Read the model definition and answer for the solid it produces. Units are mm, in the model's axes. A direction names the side the tool comes from. Coordinates: 2 decimals unless noted, no trailing zeros. Loops run counter-clockwise (first coordinate to the right, second up) from the corner with the lowest first, then second, coordinate; pieces in that order, holes last. Notation, with made-up numbers: (89, 7) - (119, 7) arc R23 ccw to (119, 17) - close; hole circle Ø6 at (53.5, -19.5). An arc over 180 degrees is marked (long way). Use one line per item in the form item = value. Start each with the question number.
1) A cutting plane is placed at D-D (y = -2.25). Give the vertices of the cut face in (x, z), and give its area (3 significant figures).
2) Which of the six approach directions +Z, -Z, +X, -X, +Y, -Y give full straight-line access (tool end or side, diameter ignored) to faces 4 (the face through (0.1, -9.9, 6.1)), 5 (the face through (15, -10, 0)), 6 (the face through (12.37, -8.606, -9.014)), 7 (the face through (11.2, -11.2, 7))?
3) A cutting plane is placed at B-B (x = 10). Give the vertices of the cut face in (y, z), and give its area (4 significant figures).
4) The mould has two halves that part along Y. Classify faces 1 (the face through (8, -20, -2)), 2 (the face through (7.61, -8.64, -9.01)), 3 (the face through (-6.97, -9.86, -7.17)): released by +Y, released by -Y, zero draft, split by the parting line, or undercut.
5) Consider line 1 (Y direction, x = 10, z = -2.75); line 2 (X direction, y = -10, z = -3); line 3 (Z direction, x = -8, y = -6.5). Determine where each line is inside the solid, lowest interval first.
6) A cutting plane is placed at A-A (z = 2.5). Give the vertices of the cut face in (x, y), and give its area (3 significant figures).
7) Each of these flat-tipped pins is pushed along its axis until it touches: P1, Ø1.6, axis at x = 10, z = -9, coming from the +Y side; P2, Ø1.6, axis at x = 10.5, y = -11, coming from the +Z side; P3, Ø2, axis at x = 24, y = -12, coming from the -Z side; P4, Ø3, axis at x = -8.5, y = -6.5, coming from the -Z side. Where does it stop, or does it pass through?
8) A cutting plane is placed at C-C (x = 1). Give the vertices of the cut face in (y, z).
from build123d import *

# Parameters (mm, degrees)
F0_R      = 6.1
F1_DEPTH  = 20
F3_R      = 1.5
F4_DEPTH  = 25
F5_DEPTH  = 25
F6_R      = 5
F7_DEPTH  = 10
F8_R      = 2.75
F8_R_2    = 1.5
F9_DEPTH  = 3
F10_R     = 1.5
F11_DEPTH = 2


with BuildPart() as f1:
    # F0 (on Front) → F1 (new body)
    with BuildSketch(Plane.XZ):
        with BuildLine():
            ThreePointArc((0, 10), (7.0710678119, 7.0710678119), (10, 0))
            ThreePointArc((10, 0), (7.0710678119, -7.0710678119), (0, -10))
            Line((0, -10), (20, -10))
            Line((20, -10), (20, 10))
            Line((20, 10), (0, 10))
        make_face()
        with BuildLine():
            ThreePointArc((0, -10), (7.0710678119, -7.0710678119), (10, 0))
            ThreePointArc((10, 0), (7.0710678119, 7.0710678119), (0, 10))
            ThreePointArc((0, 10), (-10, 0), (0, -10))
        make_face()
        Circle(F0_R, mode=Mode.SUBTRACT)
    extrude(amount=F1_DEPTH)

    # F3 (on face) → F4 (cut)
    with BuildSketch(Plane.XY.offset(10)):
        with Locations((10, -10)):
            Circle(F3_R)
    extrude(amount=-F4_DEPTH, mode=Mode.SUBTRACT)

    # F2 (on face) → F5 (cut)
    with BuildSketch(Plane.XZ.offset(20)):
        with BuildLine():
            Line((-9.9874921777, 0.5), (-17.8410350345, 0.5))
            Line((-17.8410350345, 0.5), (-17.8410350345, -0.5))
            Line((-17.8410350345, -0.5), (-9.9874921777, -0.5))
            ThreePointArc((-9.9874921777, -0.5), (-10, 0), (-9.9874921777, 0.5))
        make_face()
        with BuildLine():
            Line((-6.0794736614, 0.5), (-9.9874921777, 0.5))
            ThreePointArc((-9.9874921777, 0.5), (-10, 0), (-9.9874921777, -0.5))
            Line((-9.9874921777, -0.5), (-6.0794736614, -0.5))
            ThreePointArc((-6.0794736614, -0.5), (-6.1, 0), (-6.0794736614, 0.5))
        make_face()
        with BuildLine():
            Line((15, 0.5), (6.0794736614, 0.5))
            ThreePointArc((6.0794736614, 0.5), (6.0948662551, 0.2502105766), (6.1, 0))
            ThreePointArc((6.1, 0), (6.0948662551, -0.2502105766), (6.0794736614, -0.5))
            Line((6.0794736614, -0.5), (15, -0.5))
            Line((15, -0.5), (15, 0.5))
        make_face()
    extrude(amount=-F5_DEPTH, mode=Mode.SUBTRACT)

    # F6 (on face) → F7 (join)
    with BuildSketch(Plane.YZ.offset(20)):
        with Locations((-10, 0)):
            Circle(F6_R)
    extrude(amount=F7_DEPTH)

    # F8 (on face) → F9 (cut)
    with BuildSketch(Plane.XY.offset(10)):
        with Locations((10, -10)):
            Circle(F8_R)
        with Locations((10, -10)):
            Circle(F8_R_2, mode=Mode.SUBTRACT)
    extrude(amount=-F9_DEPTH, mode=Mode.SUBTRACT)

    # F10 (on face) → F11 (cut)
    with BuildSketch(Plane(origin=(0, 0, -10), x_dir=(1, 0, 0), z_dir=(0, 0, -1))):
        Polygon((11.5877132403, 12.75), (8.4122867597, 12.75), (6.8245735195, 10), (8.4122867597, 7.25), (11.5877132403, 7.25), (13.1754264805, 10), align=None)
        with Locations((10, 10)):
            Circle(F10_R, mode=Mode.SUBTRACT)
    extrude(amount=-F11_DEPTH, mode=Mode.SUBTRACT)


solid = f1.part
Found:
q1.outline = (-9.99, -0.5) arc R10 ccw to (0, -10) - (20, -10) - (20, 10) - (0, 10) arc R10 ccw to (-9.99, 0.5) - (-6.08, 0.5) arc R6.1 cw to (6.08, 0.5) - (15, 0.5) - (15, -0.5) - (6.08, -0.5) arc R6.1 cw to (-6.08, -0.5) - close
q1.area = 427 mm^2
q2.face_4 = +Y, -Y
q2.face_5 = -X, +Y, -Y
q2.face_6 = -Z
q2.face_7 = +Z
q3.outline = (-20, -10) - (-12.75, -10) - (-12.75, -8) - (-11.5, -8) - (-11.5, -0.5) - (-20, -0.5) - close; (-20, 0.5) - (-11.5, 0.5) - (-11.5, 7) - (-12.75, 7) - (-12.75, 10) - (-20, 10) - close; (-8.5, -8) - (-7.25, -8) - (-7.25, -10) - (0, -10) - (0, -0.5) - (-8.5, -0.5) - close; (-8.5, 0.5) - (0, 0.5) - (0, 10) - (-7.25, 10) - (-7.25, 7) - (-8.5, 7) - close
q3.area = 310.5 mm^2
q4.face_1 = released by -Y
q4.face_2 = undercut
q4.face_3 = zero draft
q5.line_1 = -20 to -11.5, -8.5 to 0
q5.line_2 = -9.54 to -5.31, 5.31 to 8.5, 11.5 to 30
q5.line_3 = -6 to -0.5, 0.5 to 6
q6.outline = (-9.68, -20) - (-5.56, -20) - (-5.56, 0) - (-9.68, 0) - close; (5.56, -20) - (20, -20) - (20, -14.33) - (30, -14.33) - (30, -5.67) - (20, -5.67) - (20, 0) - (5.56, 0) - close; hole circle Ø3 at (10, -10)
q6.area = 451 mm^2
q7.P1 = 0
q7.P2 = 7
q7.P3 = -4.9
q7.P4 = -7.14
q8.outline = (-20, -10) - (0, -10) - (0, -6.02) - (-20, -6.02) - close; (-20, 6.02) - (0, 6.02) - (0, 10) - (-20, 10) - close
